from build123d import *

# Parameters (mm, degrees)
SKETCH_2_W                   = 90
SKETCH_2_H                   = 120
SKETCH_2_R                   = 15
EXTRUDE_1_DEPTH              = 3
SKETCH_3_W                   = 90
SKETCH_3_H                   = 120
EXTRUDE_2_DEPTH              = 1
SKETCH_8_R                   = 3
EXTRUDE_5_DEPTH              = 3.5
SKETCH_10_R                  = 2
CUT_EXTRUDE_2_DEPTH          = 3.1
HOLE_WIZARD_M3_3_D           = 3.4
HOLE_WIZARD_M3_3_CSINK_D     = 6.72
HOLE_WIZARD_M3_3_CSINK_ANGLE = 90
FILLET_2_R                   = 5
FILLET_3_R                   = 5
FILLET_4_R                   = 5
FILLET_5_R                   = 5
FILLET_6_R                   = 5
FILLET_7_R                   = 5
FILLET_8_R                   = 5
FILLET_9_R                   = 5
FILLET_10_R                  = 1
SKETCH_16_R                  = 3.5
SKETCH_16_R_2                = 4
CUT_EXTRUDE_3_DEPTH          = 3


with BuildPart() as part:
    # Sketch 2 → Extrude 1 (new body)
    with BuildSketch(Plane(origin=(0, 0, 0), x_dir=(1, 0, 0), z_dir=(0, 1, 0))):
        Rectangle(SKETCH_2_W, SKETCH_2_H)
        with Locations(Location((0, 40, 0), (0, 0, 270))):
            Circle(SKETCH_2_R, mode=Mode.SUBTRACT)
    extrude(amount=EXTRUDE_1_DEPTH)



with BuildPart() as body_2:
    # Sketch 3 → Extrude 2 (new body)
    with BuildSketch(Plane.XZ):
        Rectangle(SKETCH_3_W, SKETCH_3_H)
        Polygon((-42, -50), (-42, 50), (-35, 50), (-35, 57), (35, 57), (35, 50), (42, 50), (42, -50), (35, -50), (35, -57), (-35, -57), (-35, -50), align=None, mode=Mode.SUBTRACT)
    extrude(amount=EXTRUDE_2_DEPTH)


with BuildPart() as part_1:
    add(part.part)

    add(body_2.part)  # Extrude 5 merges body 2
    # Sketch 8 → Extrude 5 (add)
    with BuildSketch(Plane.XZ):
        with BuildLine():
            Line((-5.916079783, -57), (5.916079783, -57))
            ThreePointArc((5.916079783, -57), (0, -22), (-5.916079783, -57))
        make_face()
        with Locations(Location((0, -40, 0), (0, 0, 270))):
            Circle(SKETCH_8_R, mode=Mode.SUBTRACT)
    extrude(amount=EXTRUDE_5_DEPTH)

    # Sketch 10 → Cut-Extrude 2 (cut)
    with BuildSketch(Plane(origin=(0, 0, 0), x_dir=(1, 0, 0), z_dir=(0, 1, 0))):
        with Locations(Location((0, 30, 0), (0, 0, 270))):
            Circle(SKETCH_10_R)
        with Locations(Location((10, 39.837399549, 0), (0, 0, 270))):
            Circle(SKETCH_10_R)
        with Locations(Location((0, 50, 0), (0, 0, 270))):
            Circle(SKETCH_10_R)
        with Locations(Location((-10, 40, 0), (0, 0, 270))):
            Circle(SKETCH_10_R)
    extrude(amount=-CUT_EXTRUDE_2_DEPTH, mode=Mode.SUBTRACT)

    # Hole Wizard M3 _3 (through all)
    with Locations(Plane(origin=(0, 3, 0), x_dir=(1, 0, 0), z_dir=(0, 1, 0))):
        with Locations((-40, -55), (-40, 55), (40, 55), (40, -55)):
            CounterSinkHole(HOLE_WIZARD_M3_3_D / 2, HOLE_WIZARD_M3_3_CSINK_D / 2, counter_sink_angle=HOLE_WIZARD_M3_3_CSINK_ANGLE)

    # Fillet 2
    fillet_2_edges = [part_1.edges().sort_by_distance(p)[0] for p in [
        (35, -0.5, -50),
    ]]
    fillet(fillet_2_edges, radius=FILLET_2_R)

    # Fillet 3
    fillet_3_edges = [part_1.edges().sort_by_distance(p)[0] for p in [
        (35, -0.5, 50),
    ]]
    fillet(fillet_3_edges, radius=FILLET_3_R)

    # Fillet 4
    fillet_4_edges = [part_1.edges().sort_by_distance(p)[0] for p in [
        (-35, -0.5, 50),
    ]]
    fillet(fillet_4_edges, radius=FILLET_4_R)

    # Fillet 5
    fillet_5_edges = [part_1.edges().sort_by_distance(p)[0] for p in [
        (-35, -0.5, -50),
    ]]
    fillet(fillet_5_edges, radius=FILLET_5_R)

    # Fillet 6
    fillet_6_edges = [part_1.edges().sort_by_distance(p)[0] for p in [
        (-45, 1, -60),
    ]]
    fillet(fillet_6_edges, radius=FILLET_6_R)

    # Fillet 7
    fillet_7_edges = [part_1.edges().sort_by_distance(p)[0] for p in [
        (45, 1, -60),
    ]]
    fillet(fillet_7_edges, radius=FILLET_7_R)

    # Fillet 8
    fillet_8_edges = [part_1.edges().sort_by_distance(p)[0] for p in [
        (45, 1, 60),
    ]]
    fillet(fillet_8_edges, radius=FILLET_8_R)

    # Fillet 9
    fillet_9_edges = [part_1.edges().sort_by_distance(p)[0] for p in [
        (-45, 1, 60),
    ]]
    fillet(fillet_9_edges, radius=FILLET_9_R)

    # Fillet 10
    fillet_10_edges = [part_1.edges().sort_by_distance(p)[0] for p in [
        (-45, 3, 0),
        (-43.535533906, 3, -58.535533906),
        (0, 3, -60),
        (43.535533906, 3, -58.535533906),
        (45, 3, 0),
        (43.535533906, 3, 58.535533906),
        (0, 3, 60),
        (-43.535533906, 3, 58.535533906),
    ]]
    fillet(fillet_10_edges, radius=FILLET_10_R)

    # Fillet 11: read off the stored shape, not the designer's step
    # Fillet 11 outline → Fillet 11 (revolve, cut)
    with BuildSketch(Plane.XY.offset(-40)):
        with BuildLine():
            Line((18, -3.5), (18, -1.5))
            ThreePointArc((18, -1.5), (17.414213562, -2.914213562), (16, -3.5))
            Line((16, -3.5), (18, -3.5))
        make_face()
    revolve(axis=Axis((0, 0, -40), (0, 1, 0)), mode=Mode.SUBTRACT)

    # Sketch 16 → Cut-Extrude 3 (cut)
    with BuildSketch(Plane(origin=(0, 3, 0), x_dir=(1, 0, 0), z_dir=(0, 1, 0))):
        with Locations(Location((-14.923003693, -24.181999786, 0), (0, 0, 270))):
            Circle(SKETCH_16_R)
        with Locations(Location((15.276985626, -24.181999786, 0), (0, 0, 270))):
            Circle(SKETCH_16_R_2)
    extrude(amount=-CUT_EXTRUDE_3_DEPTH, mode=Mode.SUBTRACT)


solid = part_1.part
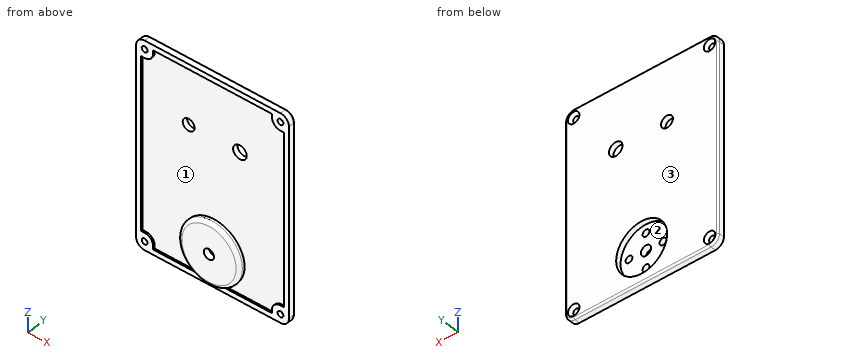
CAD build for the part. Positions are in the model's coordinates, mm. Face numbers are marked on the shaded views. Round coordinates to 2 decimals unless told otherwise and drop trailing zeros. Order: outer loops, then holes, each group sorted by start corner. A loop starts at its lowest first (then second) coordinate and runs counter-clockwise, first axis right, second up. Notation, with made-up numbers: (7, 54) -> (17, 54) arc R5 ccw to (17, 59) -> close; hole circle Ø8 at (74.5, -7). An arc over 180 degrees is marked (long way). Write item = value, one per line. Start each with the question number.
(1) Pull direction X, two halves, no side cores. Call the marked faces 1, 2 and 3: released by +X, released by -X, zero draft, split by the parting line, or undercut.
(2) Cut at B-B, the plane x = 28. List the corners of the cut face in (y, z).
(3) Probe line 1 (X direction, y = -0.75, z = -40); line 2 (X direction, y = 1.95, z = -40); line 3 (Z direction, x = -40, y = 0.75). List the from-to ranges inside material, lowest first. Write a range as [from, to].
(4) Cut at A-A, the plane z = -19.5. List the corners of the cut face in (x, y), then the cut area to 3 significant figures.
(5) Pin check, flat tips, straight feed: P1, Ø4, axis at x = -40, z = 55, coming from the -Y side; P2, Ø1.1, axis at x = 41.5, y = -0.5, coming from the +Z side; P3, Ø0.8, axis at x = 41, y = -0.5, coming from the -Z side; P4, Ø2, axis at x = 40, z = 55, coming from the -Y side. Stop position of each tip, or through.
Model answer:
q1.face_1 = undercut
q1.face_2 = undercut
q1.face_3 = zero draft
q2.outline = (-1, -60) -> (2, -60) arc R1 ccw to (3, -59) -> (3, 59) arc R1 ccw to (2, 60) -> (-1, 60) -> (-1, 57) -> (0, 57) -> (0, -57) -> (-1, -57) -> close
q3.line_1 = [-45, -42], [-18, -12], [-8, -3], [3, 8.01], [11.99, 18], [42, 45]
q3.line_2 = [-45, -15], [15, 45]
q3.line_3 = [-60, -56.7], [-53.3, 53.3], [56.7, 60]
q4.outline = (-45, -1) -> (-42, -1) -> (-42, 0) -> (42, 0) -> (42, -1) -> (45, -1) -> (45, 2) arc R1 ccw to (44, 3) -> (-44, 3) arc R1 ccw to (-45, 2) -> close
q4.area = 276 mm2
q5.P1 = -1
q5.P2 = 59.91
q5.P3 = -59.96
q5.P4 = through
